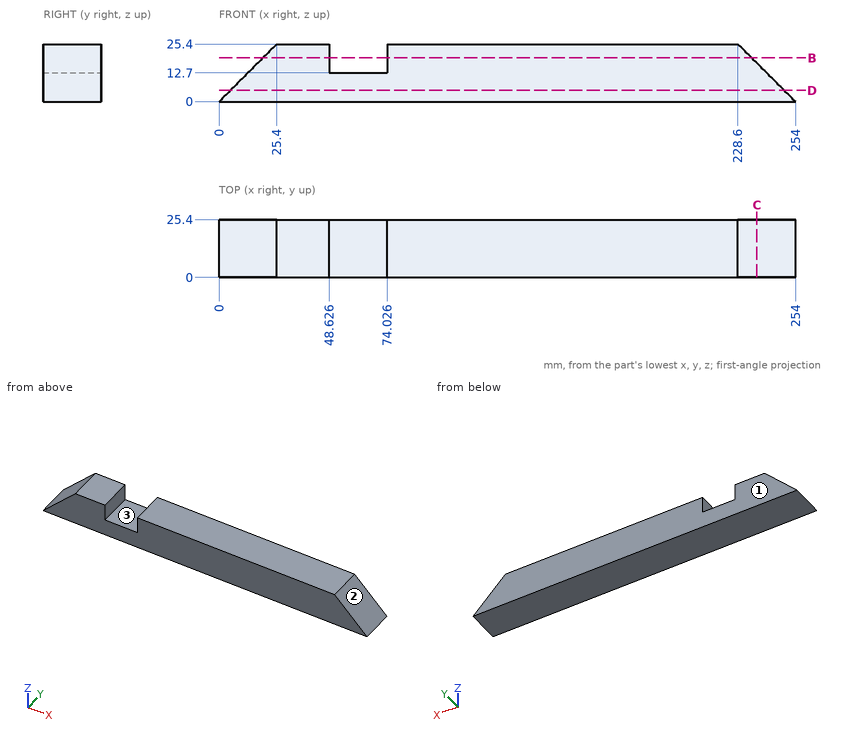
Answer from the drawing. Dimensions are ordinates in mm from the lowest x, y and z of the part. Round coordinates to 2 decimals unless told otherwise and drop trailing zeros. Order: outer loops, then holes, each group sorted by start corner. A loop starts at its lowest first (then second) coordinate and runs counter-clockwise, first axis right, second up. Notation, with made-up numbers: (34, 79.5) - (83, 79.5) arc R19 cw to (83, 95.5) - close; hole circle Ø3 at (-32, 57). An arc over 180 degrees is marked (long way). Put each result on its own line as item: value. Start each with the question number.
(1) Find section C-C (x = 237). Give the vertices of the cut face in (y, z).
(2) Straight lines are drawn through the part: probe 1 along X at (y, z) = (2, 19.5) (1 decimal); probe 2 along X at (y, z) = (19, 24) (1 decimal); probe 3 along X at (y, z) = (22.25, 1.5). For each, find the intervals that lie inside material, in ascending order. Write a range as from..to.
(3) Determine the mould class of the marked faces 1, 2 and 3 for opening direction X: released by +X, released by -X, zero draft, split by the parting line, or undercut.
(4) Find section D-D (z = 5). Give the vertices of the cut face in (x, y).
(5) Given P1, Ø12, axis at y = 3.5, z = 8, coming from the -X side; P2, Ø1.5, axis at x = 68.5, y = 8, coming from the +Z side; P3, Ø12, axis at y = 5, z = 12, coming from the +X side, each flat-ended and moving along its own axis, determine where each tip first touches the part or whether it passes through.
(6) Find section B-B (z = 19.25). Give the vertices of the cut face in (x, y), plus the area to 3 significant figures.
Reply:
1. outline: (0, 0) - (25.4, 0) - (25.4, 17) - (0, 17) - close
2. probe 1: 19.5..48.6, 74..234.5
2. probe 2: 24..48.6, 74..230
2. probe 3: 1.5..252.5
3. face 1: zero draft
3. face 2: released by +X
3. face 3: undercut
4. outline: (5, 0) - (249, 0) - (249, 25.4) - (5, 25.4) - close
5. P1: x = 2
5. P2: z = 12.7
5. P3: x = 248
6. outline: (19.25, 0) - (48.63, 0) - (48.63, 25.4) - (19.25, 25.4) - close; (74.03, 0) - (234.75, 0) - (234.75, 25.4) - (74.03, 25.4) - close
6. area: 4,830 mm^2
